```python
from build123d import *

# Parameters (mm, degrees)
SKETCH_1_R          = 26
EXTRUDE_1_DEPTH     = 5
SKETCH_2_R          = 7.5
SKETCH_2_R_2        = 2.55
EXTRUDE_2_DEPTH     = 15
SKETCH_4_R          = 1.6
CUT_EXTRUDE_1_DEPTH = 20
SKETCH_6_R          = 40.158600147
EXTRUDE_4_DEPTH     = 5
SKETCH_7_R          = 40.158600147
SKETCH_7_W          = 52
SKETCH_7_H          = 52
CUT_EXTRUDE_2_DEPTH = 5
SKETCH_8_W          = 6
SKETCH_8_H          = 42
EXTRUDE_5_DEPTH     = 45
SKETCH_9_R          = 11.5
SKETCH_9_R_2        = 1.6
CUT_EXTRUDE_3_DEPTH = 10
FILLET_1_R          = 5
FILLET_2_R          = 3


with BuildPart() as part:
    # 草图1 → 凸台-拉伸1 (new body)
    with BuildSketch(Plane.XY):
        with Locations((-2.038900501, 7.884914675)):
            Circle(SKETCH_1_R)
    extrude(amount=EXTRUDE_1_DEPTH)

    # 草图2 → 凸台-拉伸2 (add)
    with BuildSketch(Plane.XY.offset(5)):
        with Locations((-2.038900501, 7.884914675)):
            Circle(SKETCH_2_R)
        with Locations((-2.038900501, 7.884914675)):
            Circle(SKETCH_2_R_2, mode=Mode.SUBTRACT)
    extrude(amount=EXTRUDE_2_DEPTH)

    # 草图4 → 切除-拉伸1 (cut)
    with BuildSketch(Plane.ZY.offset(28.038900501)):
        with Locations((12.5, 7.884914675)):
            Circle(SKETCH_4_R)
    extrude(amount=-CUT_EXTRUDE_1_DEPTH, mode=Mode.SUBTRACT)

    # 草图6 → 凸台-拉伸4 (add)
    with BuildSketch(Plane(origin=(0, 0, 0), x_dir=(-1, 0, 0), z_dir=(0, 0, -1))):
        with Locations((2.038900501, 7.884914675)):
            Circle(SKETCH_6_R)
    extrude(amount=-EXTRUDE_4_DEPTH)

    # 草图7 → 切除-拉伸2 (cut)
    with BuildSketch(Plane(origin=(0, 0, 0), x_dir=(-1, 0, 0), z_dir=(0, 0, -1))):
        with Locations((2.038900501, 7.884914675)):
            Circle(SKETCH_7_R)
        with Locations((2.038900501, 7.884914675)):
            Rectangle(SKETCH_7_W, SKETCH_7_H, mode=Mode.SUBTRACT)
    extrude(amount=-CUT_EXTRUDE_2_DEPTH, mode=Mode.SUBTRACT)

    # 草图8 → 凸台-拉伸5 (add)
    with BuildSketch(Plane(origin=(0, 0, 0), x_dir=(-1, 0, 0), z_dir=(0, 0, -1))):
        with Locations((-5.961099499, 7.884914675)):
            Rectangle(SKETCH_8_W, SKETCH_8_H)
    extrude(amount=EXTRUDE_5_DEPTH)

    # 草图9 → 切除-拉伸3 (cut)
    with BuildSketch(Plane(origin=(8.961099499, 0, 0), x_dir=(0, 0, -1), z_dir=(1, 0, 0))):
        with Locations((24, 7.884914675)):
            Circle(SKETCH_9_R)
        with Locations((39.5, 23.384914675)):
            Circle(SKETCH_9_R_2)
        with Locations((8.5, -7.615085325)):
            Circle(SKETCH_9_R_2)
        with Locations((39.5, -7.615085325)):
            Circle(SKETCH_9_R_2)
        with Locations((8.5, 23.384914675)):
            Circle(SKETCH_9_R_2)
    extrude(amount=-CUT_EXTRUDE_3_DEPTH, mode=Mode.SUBTRACT)

    # 圆角1
    fillet_1_edges = [part.edges().sort_by_distance(p)[0] for p in [
        (5.961099499, -13.115085325, -45),
        (5.961099499, 28.884914675, -45),
    ]]
    fillet(fillet_1_edges, radius=FILLET_1_R)

    # 圆角2
    fillet_2_edges = [part.edges().sort_by_distance(p)[0] for p in [
        (8.961099499, 7.884914675, 0),
        (5.961099499, -13.115085325, 0),
        (2.961099499, 7.884914675, 0),
        (5.961099499, 28.884914675, 0),
        (-9.538900501, 7.884914675, 5),
    ]]
    fillet(fillet_2_edges, radius=FILLET_2_R)


solid = part.part
```
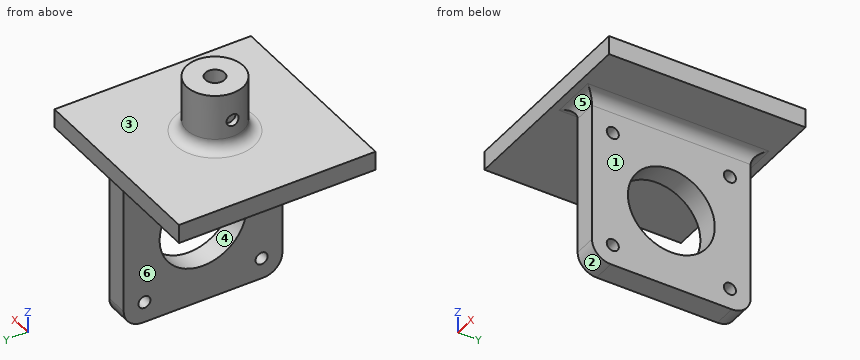
Model file for the job. Use its own axes, mm. Face numbers are marked on the shaded views. A direction names the side the tool comes from. Coordinates: 2 decimals unless noted, no trailing zeros. Loops run counter-clockwise (first coordinate to the right, second up) from the corner with the lowest first, then second, coordinate; pieces in that order, holes last. Notation, with made-up numbers: M 81.5,4.5 L 90.5,4.5 A18 cw 90.5,33.5 Z; hole C 48.25,9.5 d6. An arc over 180 degrees is marked long. Use CSV: the item, a comma, the result in double quotes. Start each with the question number.
1. Tool access for the marked faces 1, 2 and 3: list every direction of +Z, -Z, +X, -X, +Y, -Y with a clear straight run to the whole face (end or side of a thin tool).
2. Two-plate mould, pull along Z, no slides. Class the marked faces 4, 5 and 6: pulls with the +Z half, pulls with the -Z half, needs draft (parallel to the pull), parting line crosses it, or undercut.
3. Band-saw the part on D-D, the plane x = -23.5. List the corners of the cut face in (y, z).
4. Band-saw the part on C-C, the plane y = -11. List the corners of the cut face in (x, z).
5. Band-saw the part on A-A, the plane z = -8.5. List the corners of the cut face in (x, y), then the cut area to 3 significant figures.
6. Probe probe 1 along Y at (x, z) = (4.3, -39.5); probe 2 along Z at (x, y) = (4.5, 24.5); probe 3 along Y at (x, z) = (6, -39). List the from-to ranges inside material, lowest first. Write a range as [from, to].
7. Flat gauge pins, fed straight in: pin 1 (2.5 mm diameter, centred on y = -7.62, z = -8.5, fed in from -X); pin 2 (2.5 mm diameter, centred on x = -2.5, y = 7.5, fed in from +Z); pin 3 (1 mm diameter, centred on y = 8.5, z = 12, fed in from -X); pin 4 (3 mm diameter, centred on x = 0.5, y = -1.5, fed in from -Z). Where does each tip first touch, or does it go through?
8. Band-saw the part on B-B, the plane z = -24. List the corners of the cut face in (x, y), then the cut area to 3 significant figures.
Entries:
1,face 1,"-Z, +X, +Y, -Y"
1,face 2,"-Z, +X, -X, -Y"
1,face 3,"+Z"
2,face 4,"undercut"
2,face 5,"pulls with the -Z half"
2,face 6,"needs draft"
3,outline,"M -18.12,0 L 33.88,0 L 33.88,5 L -18.12,5 Z"
4,outline,"M -28.04,0 L -0.04,0 A3 cw 2.96,-3 L 2.96,-44.08 L 8.96,-44.08 L 8.96,-3 A3 cw 11.96,0 L 23.96,0 L 23.96,5 L -28.04,5 Z"
5,outline,"M 2.96,-13.12 L 8.96,-13.12 L 8.96,-9.22 L 2.96,-9.22 Z; M 2.96,-6.02 L 8.96,-6.02 L 8.96,21.78 L 2.96,21.78 Z; M 2.96,24.98 L 8.96,24.98 L 8.96,28.88 L 2.96,28.88 Z"
5,area,"214 mm2"
6,probe 1,"y = [-13.12, -9.22], [-6.02, 21.78], [24.98, 28.88]"
6,probe 2,"z = [-44.96, -40.65], [-38.35, -9.65], [-7.35, 5]"
6,probe 3,"y = [-13.12, -9.13], [-6.1, 21.87], [24.9, 28.88]"
7,pin 1,"passes through"
7,pin 2,"stops at z = 5"
7,pin 3,"stops at x = -8.04"
7,pin 4,"stops at z = -0.8"
8,outline,"M 2.96,-13.12 L 8.96,-13.12 L 8.96,-3.62 L 2.96,-3.62 Z; M 2.96,19.38 L 8.96,19.38 L 8.96,28.88 L 2.96,28.88 Z"
8,area,"114 mm2"
